Could you check a few things on this model? Use its own coordinates, in mm. Face numbers are marked on the shaded views. A direction names the side the tool comes from. Coordinates: 2 decimals unless noted, no trailing zeros. Write each loop counter-clockwise with the first axis right and the second up, starting at its lowest first coordinate (ties: lowest second). Pieces come first, ordered by that corner, then holes.
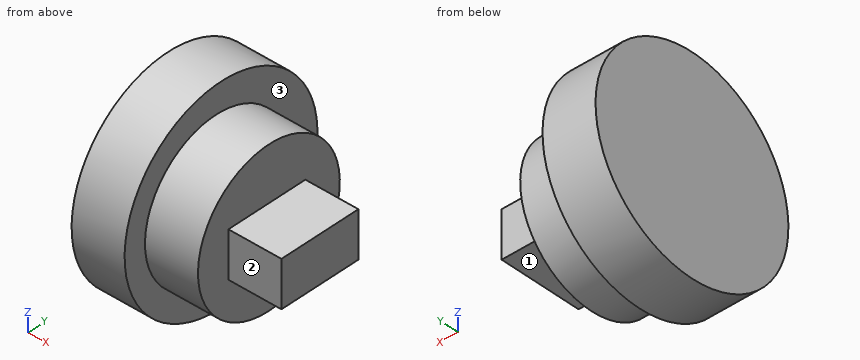
```python
from build123d import *

# Parameters (mm, degrees)
SKETCH1_R           = 19.567441598
BOSS_EXTRUDE1_DEPTH = 10
SKETCH2_R           = 14.388112676
BOSS_EXTRUDE2_DEPTH = 10
SKETCH3_W           = 8.717473042
SKETCH3_H           = 15.61355637
BOSS_EXTRUDE3_DEPTH = 10


with BuildPart() as part:
    # Sketch1 → Boss-Extrude1 (new body)
    with BuildSketch(Plane(origin=(0, 0, 0), x_dir=(0, 0, -1), z_dir=(1, 0, 0))):
        with Locations((0, 1.041985539)):
            Circle(SKETCH1_R)
    extrude(amount=BOSS_EXTRUDE1_DEPTH)

    # Sketch2 → Boss-Extrude2 (add)
    with BuildSketch(Plane(origin=(10, 0, 0), x_dir=(0, 0, -1), z_dir=(1, 0, 0))):
        Circle(SKETCH2_R)
    extrude(amount=BOSS_EXTRUDE2_DEPTH)

    # Sketch3 → Boss-Extrude3 (add)
    with BuildSketch(Plane(origin=(20, 0, 0), x_dir=(0, 0, -1), z_dir=(1, 0, 0))):
        with Locations((0.129497686, -0.406254906)):
            Rectangle(SKETCH3_W, SKETCH3_H)
    extrude(amount=BOSS_EXTRUDE3_DEPTH)


solid = part.part
```
1. On a 3-axis mill with a long thin cutter (end or side, diameter ignored), from which of +Z, -Z, +X, -X, +Y, -Y can I reach the whole of each face in a straight line? I mean the marked faces 1, 2 and 3. Say none if no direction works.
Verdict:
face 1: -Z, +X, +Y, -Y
face 2: +Z, -Z, +X, -Y
face 3: +X
2. I want a section at A-A on y = -5. Please give me the cut outline in (x, z), plus the area to 3 significant figures.
Verdict:
outline: (0, -18.61) - (10, -18.61) - (10, -13.49) - (20, -13.49) - (20, -4.49) - (30, -4.49) - (30, 4.23) - (20, 4.23) - (20, 13.49) - (10, 13.49) - (10, 18.61) - (0, 18.61) - close
area: 729 mm2
3. I want a section at D-D on z = 0. Please give me the cut outline in (x, y).
Verdict:
outline: (0, -18.53) - (10, -18.53) - (10, -14.39) - (20, -14.39) - (20, -8.21) - (30, -8.21) - (30, 7.4) - (20, 7.4) - (20, 14.39) - (10, 14.39) - (10, 20.61) - (0, 20.61) - close
4. I want a section at B-B on z = -13. Please give me the cut outline in (x, y), plus the area to 3 significant figures.
Verdict:
outline: (0, -13.58) - (10, -13.58) - (10, -6.17) - (20, -6.17) - (20, 6.17) - (10, 6.17) - (10, 15.67) - (0, 15.67) - close
area: 416 mm2
5. I want a section at C-C on x = 26.25. Please give me the cut outline in (y, z).
Verdict:
outline: (-8.21, -4.49) - (7.4, -4.49) - (7.4, 4.23) - (-8.21, 4.23) - close
6. Please list where these lines run through material, in increasing order: line 1 along Z through (x, y) = (20.25, 2); line 2 along X through (y, z) = (-9, 6.5); line 3 along Z through (x, y) = (19.25, 0.5).
Verdict:
line 1: z = -4.49 to 4.23
line 2: x = 0 to 20
line 3: z = -14.38 to 14.38
7. For pin 1 (2 mm diameter, centred on x = 3, y = 13.5, fed in from -Z); pin 2 (6 mm diameter, centred on x = 20, y = -3, fed in from +Z); pin 3 (4.5 mm diameter, centred on x = 22.5, z = 0.5, fed in from +Y), each with a flat end and sliding along its axis, tell me the tip position at first contact or that it passes through.
Verdict:
pin 1: stops at z = -15.86
pin 2: stops at z = 14.39
pin 3: stops at y = 7.4
